Could you check a few things on this model? Use its own coordinates, in mm. Give positions to 0.01 mm unless a question says otherwise; leave off trailing zeros. Loops run counter-clockwise (first coordinate to the right, second up) from the corner with the lowest first, then second, coordinate; pieces in that order, holes last. Notation, with made-up numbers: M -36.75,-16.75 L -20.75,-16.75 A13 ccw -20.75,-12.75 Z; hole C -4.5,77.25 d5. An arc over 180 degrees is marked long. Answer in a Markdown table with one row per item. Add a question column.
1. I need wall thicknesses on line 1 along X through (y, z) = (20, 0); line 2 along Z through (x, y) = (0.5, 73); line 3 along Z through (x, y) = (2, 59). Which ranges of each line are inside material? Lowest first, please. Write a range as from..to.
2. I'm going to push flat-ended pins straight in: pin 1 Ø1 at (y, z) = (81, -1) entering from +X; pin 2 Ø2 at (x, z) = (1, 0.5) entering from +Y; pin 3 Ø6 at (x, z) = (-4, 0) entering from -Y; pin 4 Ø2 at (x, y) = (2, 48) entering from +Z. Where does each tip first touch, or does it pass through?
3. If we section it at C-C on y = 72: List the corners of the cut face in (x, z) for me, then the cut area to 3 significant figures.
4. If we section it at A-A on z = 0: List the corners of the cut face in (x, y) for me.
5. If we section it at B-B on x = 0: List the corners of the cut face in (y, z) for me, then the cut area to 3 significant figures.
6. Thinking about a two-plate mould opening in X: for faces 1 (the cylindrical face through (-4.88, 48.8, -1.08)), 2 (the cylindrical face through (0.7, 48.9, 2.2)), which applies, released by +X, released by -X, zero draft, split by the parting line, or undercut?
```python
from build123d import *
from OCP.BRepFilletAPI import BRepFilletAPI_MakeChamfer

# Parameters (mm, degrees)
SKETCH1_R           = 5
BOSS_EXTRUDE1_DEPTH = 99.126978
SKETCH2_R           = 2.310056849
CUT_EXTRUDE1_DEPTH  = 100.378859761
CHAMFER1_SIZE       = 0.291338
CHAMFER1_SIZE2      = 0.150529


with BuildPart() as part:
    # Sketch1 → Boss-Extrude1 (new body)
    with BuildSketch(Plane(origin=(0, 0, 0), x_dir=(1, 0, 0), z_dir=(0, 1, 0))):
        with Locations(Location((0, 0, 0), (0, 0, 270))):
            Circle(SKETCH1_R)
    extrude(amount=BOSS_EXTRUDE1_DEPTH)

    # Sketch2 → Cut-Extrude1 (cut, through all)
    with BuildSketch(Plane(origin=(0, 0, 0), x_dir=(1, 0, 0), z_dir=(0, 1, 0))):
        with Locations(Location((0, 0, 0), (0, 0, 270))):
            Circle(SKETCH2_R)
    extrude(amount=CUT_EXTRUDE1_DEPTH, mode=Mode.SUBTRACT)

    # Chamfer1: one chamfer whose edges measure the first distance from different faces: ONE call of the kernel's chamfer builder (chamfer() names one face for all edges)
    chamfer1_edges_1 = [part.edges().sort_by_distance(p)[0] for p in [
        (0, 0, -5),
    ]]
    chamfer1_side_1 = [part.faces().sort_by_distance(p)[0] for p in [
        (0, 0, -4.858578644),
    ]]
    chamfer1_edges_2 = [part.edges().sort_by_distance(p)[0] for p in [
        (0, 99.126978, -5),
    ]]
    chamfer1_side_2 = [part.faces().sort_by_distance(p)[0] for p in [
        (0, 49.563489, -5),
    ]]
    chamfer1 = BRepFilletAPI_MakeChamfer(part.part.solid().wrapped)
    for e in chamfer1_edges_1:
        chamfer1.Add(CHAMFER1_SIZE, CHAMFER1_SIZE2, e.wrapped, chamfer1_side_1[0].wrapped)  # the first distance lies on this face
    for e in chamfer1_edges_2:
        chamfer1.Add(CHAMFER1_SIZE, CHAMFER1_SIZE2, e.wrapped, chamfer1_side_2[0].wrapped)  # the first distance lies on this face
    add(Compound.cast(chamfer1.Shape()), mode=Mode.REPLACE)


solid = part.part
```
Results:
| question | item | result |
|---|---|---|
| 1 | line 1 | -5..-2.31, 2.31..5 |
| 1 | line 2 | -4.97..-2.26, 2.26..4.97 |
| 1 | line 3 | -4.58..-1.16, 1.16..4.58 |
| 2 | pin 1 | x = 4.97 |
| 2 | pin 2 | through |
| 2 | pin 3 | y = 0 |
| 2 | pin 4 | z = 4.9 |
| 3 | outline | C 0,0 d10; hole C 0,0 d4.62 |
| 3 | area | 61.8 mm2 |
| 4 | outline | M -5,0.15 L -4.71,0 L -2.31,0 L -2.31,99.13 L -4.85,99.13 L -5,98.84 Z; M 2.31,0 L 4.71,0 L 5,0.15 L 5,98.84 L 4.85,99.13 L 2.31,99.13 Z |
| 5 | outline | M 0,-4.71 L 0.15,-5 L 98.84,-5 L 99.13,-4.85 L 99.13,-2.31 L 0,-2.31 Z; M 0,2.31 L 99.13,2.31 L 99.13,4.85 L 98.84,5 L 0.15,5 L 0,4.71 Z |
| 5 | area | 533 mm2 |
| 6 | face 1 | split by the parting line |
| 6 | face 2 | undercut |
